from build123d import *

# Parameters (mm, degrees)
SKETCH1_R           = 5
BOSS_EXTRUDE1_DEPTH = 10
SKETCH2_R           = 5
SKETCH2_R_2         = 1.25
BOSS_EXTRUDE2_DEPTH = 10


with BuildPart() as part:
    # Sketch1 → Boss-Extrude1 (new body)
    with BuildSketch(Plane.XY):
        Circle(SKETCH1_R)
        with BuildLine():
            Line((-1.072430112, -0.899940917), (-0.831301536, -0.9))
            Line((-0.831301536, -0.9), (0.831568399, -0.9))
            Line((0.831568399, -0.9), (1.07238053, -0.899999999))
            ThreePointArc((1.07238053, -0.899999999), (0.478887909, 1.315547936), (-1.4, 0))
            ThreePointArc((-1.4, 0), (-1.315561127, -0.478851669), (-1.072430112, -0.899940917))
        make_face(mode=Mode.SUBTRACT)
    extrude(amount=BOSS_EXTRUDE1_DEPTH)

    # Sketch2 → Boss-Extrude2 (add)
    with BuildSketch(Plane.XY.offset(10)):
        Circle(SKETCH2_R)
        with Locations(Location((0, 0, 0), (0, 0, 226.053894983))):
            Circle(SKETCH2_R_2, mode=Mode.SUBTRACT)
    extrude(amount=BOSS_EXTRUDE2_DEPTH)


solid = part.part
Source: CAD feature listing. Evaluate the final solid. Frame: model axes, mm. Round coordinates to 2 decimals unless told otherwise and drop trailing zeros. Loops run counter-clockwise (first coordinate to the right, second up) from the corner with the lowest first, then second, coordinate; pieces in that order, holes last.
Q1. Mould query, pull axis X, two halves, no side actions, for faces 1 (the face through (-1.2, -1, 0)), 2 (the face through (1.005, -0.743, 14.93)), 3 (the face through (-1.08, -4.88, 9.86)). Classes: pulls with the +X half, pulls with the -X half, needs draft (parallel to the pull), parting line crosses it, or undercut.
Q2. Section C-C, the plane x = 3. Return loops of the section in (y, z).
Q3. Section B-B, the plane z = 6.25. Return loops of the section in (x, y), plus the area to 3 significant figures.
Q4. Section A-A, the plane x = 0. Return loops of the section in (y, z), plus the area to 3 significant figures.
Q5. Section D-D, the plane y = 2. Return loops of the section in (x, z).
Q6. Ray query, line 1 (Y direction, x = 0, z = 12); line 2 (Y direction, x = 0, z = 5.5); line 3 (X direction, y = -0.5, z = 14.5). Return the intervals inside material, ascending.
Q7. First-contact query: P1, Ø1, axis at x = 3, z = 15.5, coming from the -Y side; P2, Ø1.5, axis at x = 3, z = 9, coming from the -Y side. Flat tips, straight axial feed; report the tip coordinate or a pass-through.
Solutions:
1. face 1: needs draft
1. face 2: undercut
1. face 3: parting line crosses it
2. outline: (-4, 0) - (4, 0) - (4, 20) - (-4, 20) - close
3. outline: circle Ø10 at (0, 0); hole (-1.07, -0.9) - (-0.83, -0.9) - (1.07, -0.9) arc R1.4 ccw (long way) to start
3. area: 73.1 mm2
4. outline: (-5, 0) - (-0.9, 0) - (-0.9, 10) - (-1.25, 10) - (-1.25, 20) - (-5, 20) - close; (1.25, 10) - (1.4, 10) - (1.4, 0) - (5, 0) - (5, 20) - (1.25, 20) - close
4. area: 152 mm2
5. outline: (-4.58, 0) - (4.58, 0) - (4.58, 20) - (-4.58, 20) - close
6. line 1: y = -5 to -1.25, 1.25 to 5
6. line 2: y = -5 to -0.9, 1.4 to 5
6. line 3: x = -4.97 to -1.15, 1.15 to 4.97
7. P1: stops at y = -4.33
7. P2: stops at y = -4.47
